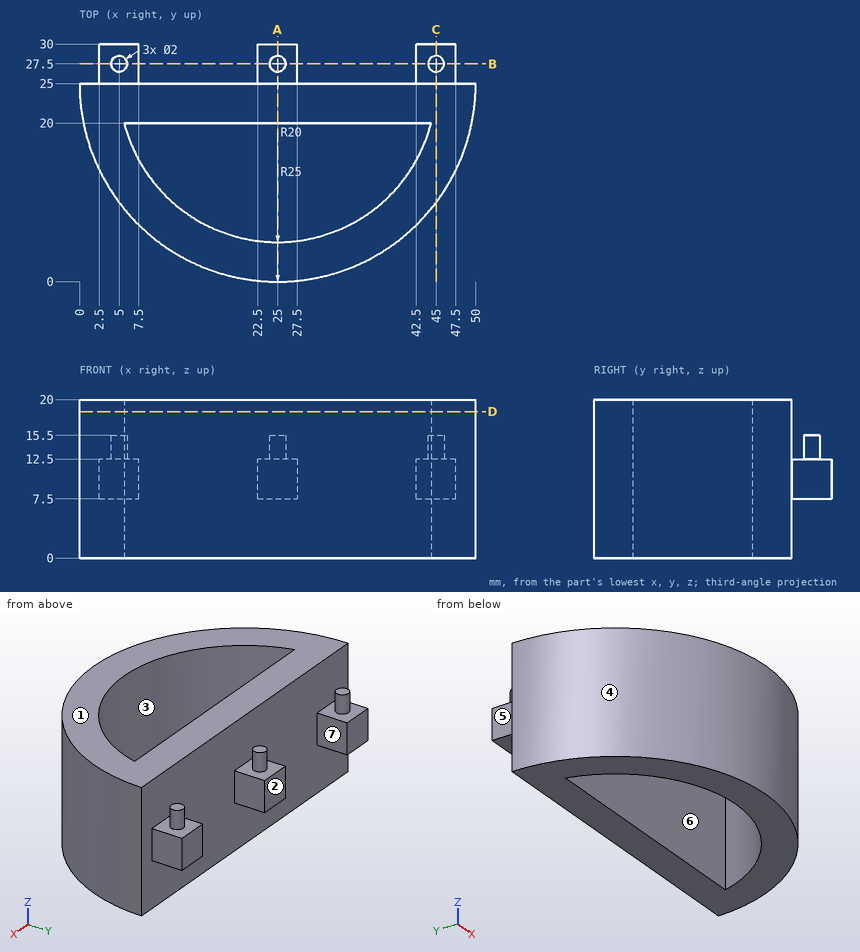
Can you work these out from the drawing? Everything is in mm from the part's minimum corner. A direction names the side the tool comes from. Give positions to 0.01 mm unless a question says otherwise; leave off trailing zeros. Write each loop counter-clockwise with the first axis right and the second up, starting at its lowest first coordinate (ties: lowest second). Pieces come first, ordered by that corner, then holes. Notation, with made-up numbers: M -26.5,22.25 L -9.5,22.25 A13 cw -9.5,29.25 Z; hole C -29,23.5 d6. An arc over 180 degrees is marked long. Answer in a Markdown table with one row per item. Add a question column.
Item 1: Please list where these lines run through material, in increasing order: L1, parallel to X at y = 27.75, z = 9.75; L2, parallel to Y at x = 24.5, z = 15.75 (3 decimals); L3, parallel to X at y = 13.5, z = 18.
Item 2: Imagine slicing it at A-A, the plane x = 25. Write out the boundary of the cut face in (y, z), plus the area to 3 significant figures.
Item 3: Imagine slicing it at B-B, the plane y = 27.5. Write out the boundary of the cut face in (x, z).
Item 4: On a 3-axis mill with a long thin cutter (end or side, diameter ignored), from which of +Z, -Z, +X, -X, +Y, -Y can I reach the whole of each face in a straight line? I mean the marked faces 5, 6 and 7. Say none if no direction works.
Item 5: Imagine slicing it at D-D, the plane z = 18.5. Write out the boundary of the cut face in (x, y).
Item 6: For pin 1 Ø6 at (x, y) = (12.5, 14.5) entering from +Z; pin 2 Ø2.5 at (x, y) = (44, 28) entering from +Z; pin 3 Ø6 at (y, z) = (7, 15.5) entering from +X; pin 4 Ø1 at (y, z) = (10.5, 5.5) entering from -X, each with a flat end and sliding along its axis, tell me the tip position at first contact or that it passes through.
Item 7: We'd pull the mould along Y, two halves only. Please class the marked faces 1, 2, 3 and 4: released by +Y, released by -Y, zero draft, split by the parting line, or undercut.
Item 8: Imagine slicing it at C-C, the plane x = 45. Write out the boundary of the cut face in (y, z).
Evaluation:
| question | item | result |
|---|---|---|
| 1 | L1 | x = 2.5 to 7.5, 22.5 to 27.5, 42.5 to 47.5 |
| 1 | L2 | y = 0.005 to 5.006, 20 to 25 |
| 1 | L3 | x = 2.8 to 8.64, 41.36 to 47.2 |
| 2 | outline | M 0,0 L 5,0 L 5,20 L 0,20 Z; M 20,0 L 25,0 L 25,7.5 L 30,7.5 L 30,12.5 L 28.5,12.5 L 28.5,15.5 L 26.5,15.5 L 26.5,12.5 L 25,12.5 L 25,20 L 20,20 Z |
| 2 | area | 231 mm² |
| 3 | outline | M 2.5,7.5 L 7.5,7.5 L 7.5,12.5 L 6,12.5 L 6,15.5 L 4,15.5 L 4,12.5 L 2.5,12.5 Z; M 22.5,7.5 L 27.5,7.5 L 27.5,12.5 L 26,12.5 L 26,15.5 L 24,15.5 L 24,12.5 L 22.5,12.5 Z; M 42.5,7.5 L 47.5,7.5 L 47.5,12.5 L 46,12.5 L 46,15.5 L 44,15.5 L 44,12.5 L 42.5,12.5 Z |
| 4 | face 5 | +Z, -Z, -X, +Y |
| 4 | face 6 | +Z, -Z |
| 4 | face 7 | +Z, -Z, +Y |
| 5 | outline | M 0,25 A25 ccw 50,25 Z; hole M 5.64,20 A20 ccw 44.36,20 Z |
| 6 | pin 1 | passes through |
| 6 | pin 2 | stops at z = 15.5 |
| 6 | pin 3 | stops at x = 45 |
| 6 | pin 4 | stops at x = 4.29 |
| 7 | face 1 | zero draft |
| 7 | face 2 | released by +Y |
| 7 | face 3 | undercut |
| 7 | face 4 | released by -Y |
| 8 | outline | M 10,0 L 25,0 L 25,7.5 L 30,7.5 L 30,12.5 L 28.5,12.5 L 28.5,15.5 L 26.5,15.5 L 26.5,12.5 L 25,12.5 L 25,20 L 10,20 Z |
